from build123d import *

# Parameters (mm, degrees)
EXTRUDE_1_DEPTH     = 225
CUT_EXTRUDE_1_DEPTH = 226.363982288
SKETCH_4_R          = 2.13
CUT_EXTRUDE_2_DEPTH = 8.5


with BuildPart() as part:
    # Sketch 1 → Extrude 1 (new body)
    with BuildSketch(Plane(origin=(0, 0, 0), x_dir=(0, 0, -1), z_dir=(1, 0, 0))):
        Polygon((9.053300859, -3.75), (9.053300859, 3.75), (3.75, 9.053300859), (-3.75, 9.053300859), (-9.053300859, 3.75), (-9.053300859, -3.75), (-3.75, -9.053300859), (3.75, -9.053300859), align=None)
    extrude(amount=EXTRUDE_1_DEPTH)

    # Sketch 2 → Cut-Extrude 1 (cut, through all)
    with BuildSketch(Plane(origin=(225, 0, 0), x_dir=(0, 0, -1), z_dir=(1, 0, 0))):
        with BuildLine():
            Line((-1.859690835, 1.859690835), (0, 3.719381669))
            Line((0, 3.719381669), (1.859690835, 1.859690835))
            ThreePointArc((1.859690835, 1.859690835), (0, -2.63), (-1.859690835, 1.859690835))
        make_face()
    extrude(amount=-CUT_EXTRUDE_1_DEPTH, mode=Mode.SUBTRACT)

    # Sketch 4 → Cut-Extrude 2 (cut)
    with BuildSketch(Plane(origin=(0, 0, 9.053300859), x_dir=(1, 0, 0), z_dir=(0, 0, -1))):
        with Locations(Location((4, 0, 0), (0, 0, 299.179768577))):
            Circle(SKETCH_4_R)
        with Locations(Location((221, 0, 0), (0, 0, 299.179768577))):
            Circle(SKETCH_4_R)
    extrude(amount=CUT_EXTRUDE_2_DEPTH, mode=Mode.SUBTRACT)


solid = part.part
Read the model definition and answer for the solid it produces. Units are mm, in the model's axes. A direction names the side the tool comes from. Coordinates: 2 decimals unless noted, no trailing zeros. Loops run counter-clockwise (first coordinate to the right, second up) from the corner with the lowest first, then second, coordinate; pieces in that order, holes last.
Q1. The mould has two halves that part along Y. Classify faces 1 (the face through (110.925, 6.439, 6.365)), 2 (the face through (218.96, 0.61, 5.35)), 3 (the face through (110.925, -6.439, -6.365)), 4 (the face through (114.08, -2.63, -0.09)): +Y half, -Y half, draft (parallel to the pull), parting line (faces both ways), or undercut.
Q2. Consider probe 1 along X at (y, z) = (0, 4); probe 2 along Z at (x, y) = (58, 0); probe 3 along Y at (x, z) = (221, 3.5). Determine where each line is inside the solid, lowest interval first.
Q3. Each of these flat-tipped pins is pushed along its axis until it touches: pin 1 Ø3.5 at (x, y) = (221, 0) entering from +Z; pin 2 Ø6 at (y, z) = (0, -6) entering from -X; pin 3 Ø1.5 at (x, z) = (64.5, -6) entering from -Y; pin 4 Ø2.5 at (x, y) = (4, 0) entering from +Z. Where does it stop, or does it pass through?
Q4. Which of the six approach directions +Z, -Z, +X, -X, +Y, -Y give full straight-line access (tool end or side, diameter ignored) to faces 5 (the face through (225, 2, 2)), 6 (the face through (1.96, 0.61, 5.35))?
Q5. The part is cut by section B-B on x = 79.5. Write down the section's boundary in (y, z).
Q6. The part is cut by section A-A on y = 0. Write down the section's boundary in (x, z), and give its area (3 significant figures).
Results below:
1. face 1: +Y half
1. face 2: undercut
1. face 3: -Y half
1. face 4: undercut
2. probe 1: x = 0 to 1.87, 6.13 to 218.87, 223.13 to 225
2. probe 2: z = -9.05 to -2.63, 2.63 to 9.05
2. probe 3: y = -9.05 to -2.13, 2.13 to 9.05
3. pin 1: stops at z = -1.96
3. pin 2: stops at x = 0
3. pin 3: stops at y = -7.55
3. pin 4: stops at z = -2.31
4. face 5: +Z, -Z, +X, +Y, -Y
4. face 6: +Z
5. outline: (-9.05, -3.75) - (-3.75, -9.05) - (3.75, -9.05) - (9.05, -3.75) - (9.05, 3.75) - (3.75, 9.05) - (-3.75, 9.05) - (-9.05, 3.75) - close; hole (1.86, -1.86) - (3.72, 0) - (1.86, 1.86) arc R2.63 ccw (long way) to start
6. outline: (0, -9.05) - (225, -9.05) - (225, -2.63) - (0, -2.63) - close; (0, 2.63) - (1.87, 2.63) - (1.87, 9.05) - (0, 9.05) - close; (6.13, 2.63) - (218.87, 2.63) - (218.87, 9.05) - (6.13, 9.05) - close; (223.13, 2.63) - (225, 2.63) - (225, 9.05) - (223.13, 9.05) - close
6. area: 2,840 mm2
